Geometry: final body of the model. Coordinates: model frame, mm. A direction names the side the tool comes from. Give positions to 0.01 mm unless a question says otherwise; leave off trailing zeros. Write each loop counter-clockwise with the first axis right and the second up, starting at its lowest first coordinate (ties: lowest second). Pieces come first, ordered by that corner, then holes.
Solid Edge part; units mm, degrees
sketch "Sketch1" plane through (0, 0, 0) normal (0, -1, 0) x (1, 0, 0)
  circle A0 centre (0, 0) radius 2.5
extrude "Protrusion1" add sketch "Sketch1" against normal blind 20
sketch "Sketch2" plane through (0, 0, 0) normal (0, -1, 0) x (1, 0, 0)
  circle A0 centre (0, 0) radius 3.5
extrude "ExtrudedProtrusion_2" add sketch "Sketch2" along normal blind 5
fillet "Round_1" radius 0.3 1 edges at (-3.5, -5, 0)
chamfer "Chamfer_1" distance 0.5 angle 45 1 edges at (-2.5, 20, 0) measured on face at (-1.6167, 20, 1.7167)
sketch "Sketch3" plane through (0, -5, 0) normal (0, -1, 0) x (1, 0, 0)
  line L0 (-0.9646, 1.6708) -> (-1.9293, 0)
  line L1 (-1.9293, 0) -> (-0.9646, -1.6708)
  line L2 (-0.9646, -1.6708) -> (0.9646, -1.6708)
  line L3 (0.9646, -1.6708) -> (1.9293, 0)
  line L4 (1.9293, 0) -> (0.9646, 1.6708)
  line L5 (0.9646, 1.6708) -> (-0.9646, 1.6708)
extrude "ExtrudedCutout_1" cut sketch "Sketch3" along normal mid plane 8
cosmetic_thread "Thread1"
Q1. Section B-B on y = 11.75. Output: boundary loops of the cut face in (x, z), plus the area to 3 significant figures.
Filled sheet:
outline: circle Ø5 at (0, 0)
area: 19.6 mm2
Q2. Pin query (flat end, axial travel): P1, Ø4, axis at x = -1.5, y = 3, coming from the -Z side; P2, Ø3, axis at x = -1.5, y = 14, coming from the +Z side. Return the tip coordinate at first contact, or that it passes through.
Filled sheet:
P1: stops at z = -2.5
P2: stops at z = 2.5
Q3. Ray query, line 1 along Y through (x, z) = (2.5, 1); line 2 along Y through (x, z) = (-1, 0); line 3 along Z through (x, y) = (1.5, 5.25). Return the intervals inside material, ascending.
Filled sheet:
line 1: y = -5 to 0
line 2: y = -1 to 20
line 3: z = -2 to 2
Q4. Section A-A on x = 0. Output: boundary loops of the cut face in (y, z), plus the area to 3 significant figures.
Filled sheet:
outline: (-5, -3.2) arc R0.3 ccw to (-4.7, -3.5) - (0, -3.5) - (0, -2.5) - (19.5, -2.5) - (20, -2) - (20, 2) - (19.5, 2.5) - (0, 2.5) - (0, 3.5) - (-4.7, 3.5) arc R0.3 ccw to (-5, 3.2) - (-5, 1.67) - (-1, 1.67) - (-1, -1.67) - (-5, -1.67) - close
area: 121 mm2
Q5. Access query for faces 1 (the flat face through (-1.4, -5, -1.4)), 2 (the flat face through (-1.454, -2.972, -0.824)), 3 (the flat face through (-2, 0, -2)). Directions: +Z, -Z, +X, -X, +Y, -Y. A direction counts if a zero-diameter tool reaches every point of the face in a straight line with its end or side. Return the directions, or none.
Filled sheet:
face 1: +Z, -Z, +X, -X, -Y
face 2: -Y
face 3: +Y
Q6. Pull-direction query (Z, two-part tool) for faces 4 (the flat face through (0, -1, 0)), 5 (the flat face through (0, 20, 0)), 6 (the cylindrical face through (-0.54, 9.61, -2.44)); classes: released by +Z, released by -Z, zero draft, split by the parting line, or undercut.
Filled sheet:
face 4: undercut
face 5: zero draft
face 6: split by the parting line
